Can you work these out from the model? Positions are in its coordinate system, mm. A direction names the side the tool comes from. Give positions to 0.01 mm unless a question says otherwise; leave off trailing zeros. Write each loop counter-clockwise with the first axis right and the second up, starting at its lowest first coordinate (ties: lowest second). Pieces come first, ordered by that corner, then holes. Notation, with made-up numbers: (24, 57.5) - (55, 57.5) arc R29 ccw to (55, 80.5) - close; hole circle Ø11 at (-12, -6). An arc over 180 degrees is marked (long way). Use a Markdown table: item, result. Add a question column.
```python
from build123d import *

# Parameters (mm, degrees)
F0_R      = 34.6399806849
F1_DEPTH  = 50.8
F2_DEPTH  = 50.8
F4_DEPTH  = 25.4
F5_DEPTH  = 50.8
F6_DEPTH  = 25.4
F7_R      = 26.5192629278
F8_DEPTH  = 25.4
F9_R      = 25.3977072723
F10_DEPTH = 25.4


with BuildPart() as f1:
    # F0 (on Front) → F1 (new body)
    with BuildSketch(Plane.XZ):
        Circle(F0_R)
    extrude(amount=F1_DEPTH)

    # F2 (add): a face of the model
    f2_faces = [f1.faces().sort_by_distance(p)[0] for p in [
        (0, -50.8, 0),
    ]]
    extrude(f2_faces, amount=F2_DEPTH)

    # F3 (on Front) → F4 (join)
    with BuildSketch(Plane.XZ):
        with BuildLine():
            Line((17.0650705695, 25.7374811918), (33.8503867388, 9.7914338112))
            ThreePointArc((33.8503867388, 9.7914338112), (47.4968674715, 40.9635553292), (17.0650705695, 25.7374811918))
        make_face()
    extrude(amount=F4_DEPTH)

    # F5 (add): a face of the model
    f5_faces = [f1.faces().sort_by_distance(p)[0] for p in [
        (7.0012928433, 0, 5.5654888529),
    ]]
    extrude(f5_faces, amount=-F5_DEPTH)

    # F6 (add): a face of the model
    f6_faces = [f1.faces().sort_by_distance(p)[0] for p in [
        (7.0012928433, 0, 5.5654888529),
    ]]
    extrude(f6_faces, amount=-F6_DEPTH)

    # F7 (on Front) → F8 (cut)
    with BuildSketch(Plane.XZ):
        Circle(F7_R)
    extrude(amount=-F8_DEPTH, mode=Mode.SUBTRACT)

    # F9 (on Front) → F10 (cut)
    with BuildSketch(Plane.XZ):
        Circle(F9_R)
    extrude(amount=-F10_DEPTH, mode=Mode.SUBTRACT)


solid = f1.part
```
Q1. Suppose I cut it at D-D (z = 0). Please give me the cut outline in (x, y), and give its area (3 significant figures).
Q2. On a 3-axis mill with a long thin cutter (end or side, diameter ignored), from which of +Z, -Z, +X, -X, +Y, -Y can I reach the whole of each face in a straight line? I mean faces 1 (the flat face through (9, 0, 6)), 2 (the flat face through (39, -50.8, 28)). Say none if no direction works.
Q3. Suppose I cut it at B-B (y = -58). Please give me the cut outline in (x, z).
Q4. Suppose I cut it at C-C (z = 28.5). Please give me the cut outline in (x, y).
Q5. I'm going to push flat-ended pins straight in: P1, Ø10, axis at x = 10, z = -23.5, coming from the +Y side; P2, Ø8, axis at y = -40.5, z = 21.5, coming from the +X side; P3, Ø8, axis at x = 43, y = -26.5, coming from the -Z side; P4, Ø5, axis at y = -86, z = -1.5, coming from the +X side. Where does each tip first touch, or does it pass through?
Q6. Suppose I cut it at A-A (x = 0). Please give me the cut outline in (y, z), and give its area (3 significant figures).
Q7. If I drill on probe 1 along Y at (x, z) = (33, 19.5); probe 2 along Z at (x, y) = (-1, -44); probe 3 along Z at (x, y) = (-2.5, -15.5), over which ranges is the centre line in solid material (lowest first)? Write a range as [from, to].
Derived:
| question | item | result |
|---|---|---|
| 1 | outline | (-34.64, -101.6) - (34.64, -101.6) - (34.64, 0) - (-34.64, 0) - close |
| 1 | area | 7,040 mm² |
| 2 | face 1 | +Z, -Z, +X, -X, +Y |
| 2 | face 2 | +Z, +X, -Y |
| 3 | outline | circle Ø69.28 at (0, 0) |
| 4 | outline | (-19.69, -101.6) - (19.69, -101.6) - (19.69, -50.8) - (53.12, -50.8) - (53.12, 0) - (-19.69, 0) - close |
| 5 | P1 | y = 0 |
| 5 | P2 | x = 52.98 |
| 5 | P3 | z = 10.19 |
| 5 | P4 | x = 34.64 |
| 6 | outline | (-101.6, -34.64) - (0, -34.64) - (0, 34.64) - (-101.6, 34.64) - close |
| 6 | area | 7,040 mm² |
| 7 | probe 1 | [-50.8, 0] |
| 7 | probe 2 | [-34.63, 34.63] |
| 7 | probe 3 | [-34.55, 34.55] |
